Check sheet for the drawn part. Datum: minimum x, y, z corner. Units: mm. A direction names the side the tool comes from. Coordinates: 2 decimals unless noted, no trailing zeros. Order: outer loops, then holes, each group sorted by start corner. A loop starts at its lowest first (then second) coordinate and runs counter-clockwise, first axis right, second up.
Q1. Cross-section at A-A, the plane z = 1.2. Record the boundary of the cut face in (x, y).
Q2. Cross-section at C-C, the plane y = 21. Record the boundary of the cut face in (x, z).
Q3. Depth check by flat-ended pin: P1, Ø2.5, axis at y = 25, z = 2, coming from the -X side; P2, Ø6.5, axis at x = 33.5, y = 8, coming from the -Z side. Enter the tip coordinate at first touch or a pass-through.
Q4. Set-up check for the marked faces 1 and 2: record each of +Z, -Z, +X, -X, +Y, -Y from which the full face is reachable in a straight line by a thin tool's end or side.
Q5. Draft check along X on the marked faces 3, 4 and 5. Enter one of: pulls with the +X half, pulls with the -X half, needs draft (parallel to the pull), parting line crosses it, or undercut.
Q6. Thickness scan on line 1 (Y direction, x = 22, z = 1.75); line 2 (X direction, y = 27.5, z = 1.35); line 3 (Z direction, x = 45, y = 3.5). Record the ranges inside material, lowest first.
Q7. Cross-section at B-B, the plane x = 33. Record the boundary of the cut face in (y, z).
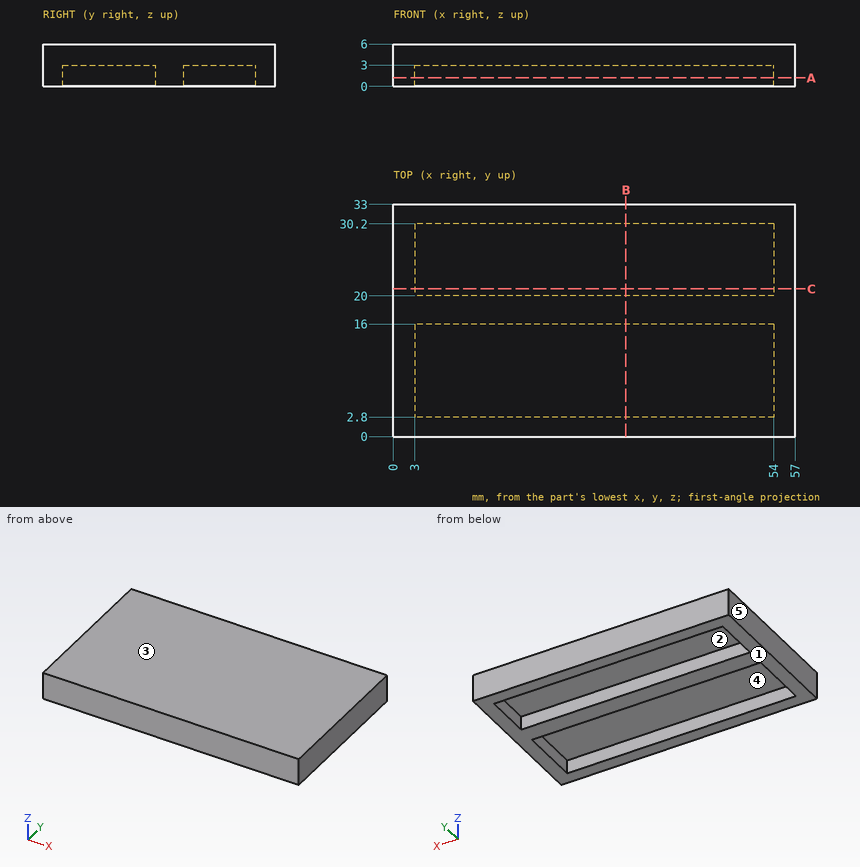
Check values:
1. outline: (0, 0) - (57, 0) - (57, 33) - (0, 33) - close; hole (3, 2.8) - (54, 2.8) - (54, 16) - (3, 16) - close; hole (3, 20) - (54, 20) - (54, 30.2) - (3, 30.2) - close
2. outline: (0, 0) - (3, 0) - (3, 3) - (54, 3) - (54, 0) - (57, 0) - (57, 6) - (0, 6) - close
3. P1: stops at x = 0
3. P2: stops at z = 3
4. face 1: -Z, +X, -X, +Y, -Y
4. face 2: -Z
5. face 3: needs draft
5. face 4: undercut
5. face 5: pulls with the -X half
6. line 1: y = 0 to 2.8, 16 to 20, 30.2 to 33
6. line 2: x = 0 to 3, 54 to 57
6. line 3: z = 3 to 6
7. outline: (0, 0) - (2.8, 0) - (2.8, 3) - (16, 3) - (16, 0) - (20, 0) - (20, 3) - (30.2, 3) - (30.2, 0) - (33, 0) - (33, 6) - (0, 6) - close
